The model under review builds one solid part; all positions refer to its coordinate system, in mm. Face numbers are marked on the shaded views. A direction names the side the tool comes from. Give positions to 0.01 mm unless a question says otherwise; leave off trailing zeros. Loops run counter-clockwise (first coordinate to the right, second up) from the corner with the lowest first, then second, coordinate; pieces in that order, holes last. Notation, with made-up numbers: M 40,11 L 90,11 A31 ccw 90,40 Z; hole C 62,78 d3. An arc over 180 degrees is marked long. Return JSON: item names as keys, results as strings.
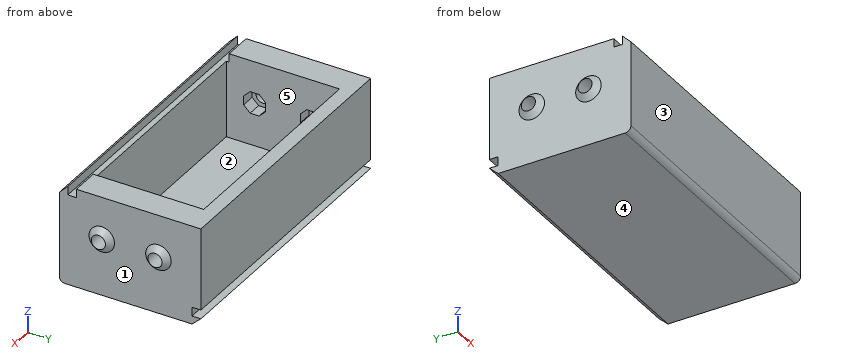
Solid Edge part; units mm, degrees
sketch "Sketch1" plane through (0, 0, 0) normal (-1, 0, 0) x (0, -1, 0)
  line L0 (25, -17.5) -> (25, 17.5)
  line L1 (25, 17.5) -> (-25, 17.5)
  line L2 (-25, 17.5) -> (-25, -17.5)
  line L3 (-25, -17.5) -> (25, -17.5)
extrude "Protrusion1" add sketch "Sketch1" along normal blind 100
sketch "Sketch2" plane through (-50, 0, 17.5) normal (0, 0, 1) x (0, 1, 0)
  line L0 (20, 45) -> (20, -45)
  line L1 (-20, -45) -> (20, -45)
  line L2 (-20, 45) -> (-20, -45)
  line L3 (-20, 45) -> (20, 45)
extrude "Cutout1" cut sketch "Sketch2" against normal blind 30
sketch "Sketch3" plane through (-5, 0, 2.5) normal (-1, 0, 0) x (0, 1, 0)
  line L0 (-20, 15) -> (20, 15)
  line L1 (20, 15) -> (20, -15)
  line L2 (20, -15) -> (-20, -15)
  line L3 (-20, -15) -> (-20, 15)
  line L4 (11.5947, -3.85) -> (8.4053, -3.85)
  line L5 (8.4053, -3.85) -> (6.15, -1.5947)
  line L6 (6.15, -1.5947) -> (6.15, 1.5947)
  line L7 (6.15, 1.5947) -> (8.4053, 3.85)
  line L8 (8.4053, 3.85) -> (11.5947, 3.85)
  line L9 (11.5947, 3.85) -> (13.85, 1.5947)
  line L10 (13.85, 1.5947) -> (13.85, -1.5947)
  line L11 (13.85, -1.5947) -> (11.5947, -3.85)
  line L12 (-11.5947, -3.85) -> (-8.4053, -3.85)
  line L13 (-8.4053, -3.85) -> (-6.15, -1.5947)
  line L14 (-6.15, -1.5947) -> (-6.15, 1.5947)
  line L15 (-6.15, 1.5947) -> (-8.4053, 3.85)
  line L16 (-8.4053, 3.85) -> (-11.5947, 3.85)
  line L17 (-11.5947, 3.85) -> (-13.85, 1.5947)
  line L18 (-13.85, 1.5947) -> (-13.85, -1.5947)
  line L19 (-13.85, -1.5947) -> (-11.5947, -3.85)
extrude "Protrusion2" add sketch "Sketch3" along normal blind 5
sketch "Sketch4" plane through (0, 0, 0) normal (1, 0, 0) x (0, 1, 0)
  circle A0 centre (-10, 2.5) radius 2.5
  circle A1 centre (10, 2.5) radius 2.5
extrude "ExtrudedProtrusion_27" add sketch "Sketch4" along normal blind 5
chamfer "Chamfer_14" distance 2 angle 45 2 edges at (0, 7.5, 2.5) (0, -12.5, 2.5)
sketch "Sketch5" plane through (-100, 0, 0) normal (-1, 0, 0) x (0, -1, 0)
  circle A0 centre (-10, 2.5) radius 2.5
  circle A1 centre (10, 2.5) radius 2.5
extrude "ExtrudedProtrusion_29" add sketch "Sketch5" along normal blind 5
chamfer "Chamfer1" distance 2 angle 45 2 edges at (-100, 10, 0) (-100, -10, 0)
sketch "Sketch6" plane through (-105, 10, 2.5) normal (-1, 0, 0) x (0, -1, 0)
  circle A0 centre (0, 0) radius 2.5
  circle A1 centre (20, 0) radius 2.5
extrude "ExtrudedCutout_41" cut sketch "Sketch6" against normal blind 159
sketch "Sketch7" plane through (-95, 0, 2.5) normal (1, 0, 0) x (0, -1, 0)
  line L0 (-20, 15) -> (20, 15)
  line L1 (20, 15) -> (20, -15)
  line L2 (20, -15) -> (-20, -15)
  line L3 (-20, -15) -> (-20, 15)
  line L4 (-11.5947, 3.85) -> (-8.4053, 3.85)
  line L5 (-8.4053, 3.85) -> (-6.15, 1.5947)
  line L6 (-6.15, 1.5947) -> (-6.15, -1.5947)
  line L7 (-6.15, -1.5947) -> (-8.4053, -3.85)
  line L8 (-8.4053, -3.85) -> (-11.5947, -3.85)
  line L9 (-11.5947, -3.85) -> (-13.85, -1.5947)
  line L10 (-13.85, -1.5947) -> (-13.85, 1.5947)
  line L11 (-13.85, 1.5947) -> (-11.5947, 3.85)
  line L12 (6.15, 1.5947) -> (6.15, -1.5947)
  line L13 (6.15, -1.5947) -> (8.4053, -3.85)
  line L14 (8.4053, -3.85) -> (11.5947, -3.85)
  line L15 (11.5947, -3.85) -> (13.85, -1.5947)
  line L16 (13.85, -1.5947) -> (13.85, 1.5947)
  line L17 (13.85, 1.5947) -> (11.5947, 3.85)
  line L18 (11.5947, 3.85) -> (8.4053, 3.85)
  line L19 (8.4053, 3.85) -> (6.15, 1.5947)
extrude "ExtrudedProtrusion_30" add sketch "Sketch7" along normal blind 5
sketch "Sketch8" plane through (0, 0, 0) normal (1, 0, 0) x (0, -1, 0)
  line L0 (-25, 11.5) -> (-21.85, 11.5)
  line L1 (-21.85, 11.5) -> (-21.85, 14.65)
  line L2 (-21.85, 14.65) -> (-25, 14.65)
  line L3 (-25, 14.65) -> (-21.85, 17.5)
  line L4 (-21.85, 17.5) -> (-21.85, 20.916)
  line L5 (-21.85, 20.916) -> (-29.169, 20.916)
  line L6 (-29.169, 20.916) -> (-29.169, 11.5)
  line L7 (-29.169, 11.5) -> (-25, 11.5)
extrude "Cutout2" cut sketch "Sketch8" against normal blind 112
fillet "Round_8" radius 2 1 edges at (-50, -25, -17.5)
sketch "Sketch9" plane through (0, 0, 0) normal (1, 0, 0) x (0, -1, 0)
  line L0 (22, -14.5) -> (22, -17.5)
  line L1 (25, -14.5) -> (22, -17.5)
  line L2 (25, -14.5) -> (26.5677, -14.5)
  line L3 (26.5677, -14.5) -> (24.562, -20.6312)
  line L4 (24.562, -20.6312) -> (19, -21.06)
  line L5 (19, -14.5) -> (19, -21.06)
  line L6 (19, -14.5) -> (22, -14.5)
extrude "ExtrudedCutout_43" cut sketch "Sketch9" against normal blind 210
1) Wall thickness on L1, parallel to Y at x = -3.5, z = 2.5; L2, parallel to Y at x = -38.5, z = 12.5; L3, parallel to X at y = 13.5, z = 8.5: over which ranges is each line inside the solid? List them lowest first. Write a range as from..to.
From the geometry:
{"L1": "-25..-12.5, -7.5..7.5, 12.5..25", "L2": "-25..-20, 20..25", "L3": "-100..-90, -10..0"}
2) Consider section C-C on z = 11.5. Write out the cut boundary in (x, y).
From the geometry:
{"outline": "M -100,-25 L 0,-25 L 0,25 L -100,25 Z; hole M -90,-20 L -10,-20 L -10,20 L -90,20 Z"}
3) Consider section B-B on x = -17. Write out the cut boundary in (y, z), then the cut area to 3 significant figures.
From the geometry:
{"outline": "M -25,-15.5 A2 ccw -23,-17.5 L 21.85,-17.5 L 25,-14.65 L 21.85,-14.65 L 21.85,-11.5 L 25,-11.5 L 25,17.5 L 20,17.5 L 20,-12.5 L -20,-12.5 L -20,14.5 L -22,14.5 L -22,17.5 L -25,14.5 Z", "area": "524 mm²"}
4) The part is to be moulded in two halves that separate along X. For the marked faces 1, 2 and 3, say which applies: released by +X, released by -X, zero draft, split by the parting line, or undercut.
From the geometry:
{"face 1": "released by +X", "face 2": "undercut", "face 3": "zero draft"}
5) Consider section D-D on y = 4. Write out the cut boundary in (x, z).
From the geometry:
{"outline": "M -100,-17.5 L 0,-17.5 L 0,17.5 L -10,17.5 L -10,-12.5 L -90,-12.5 L -90,17.5 L -100,17.5 Z"}
6) Tool access review of the marked faces 4 and 5: name each direction out of +Z, -Z, +X, -X, +Y, -Y from which nothing blocks a thin tool from reaching the whole face with its end or side.
From the geometry:
{"face 4": "-Z, +X, -X, +Y, -Y", "face 5": "+Z"}
7) Consider section A-A on y = -10. Write out the cut boundary in (x, z).
From the geometry:
{"outline": "M -102,0 L -100,-2 L -100,-17.5 L 0,-17.5 L 0,-2 L 2,0 L -5,0 L -5,-1.35 L -10,-1.35 L -10,-12.5 L -90,-12.5 L -90,-1.35 L -95,-1.35 L -95,0 Z; M -102,5 L -95,5 L -95,6.35 L -90,6.35 L -90,17.5 L -100,17.5 L -100,7 Z; M -10,6.35 L -5,6.35 L -5,5 L 2,5 L 0,7 L 0,17.5 L -10,17.5 Z"}
8) Insertion check: pin 1 (1.6 mm diameter, centred on x = -74.5, y = 23, fed in from -Z); pin 2 (5 mm diameter, centred on x = -45, y = -7.5, fed in from +Z); pin 3 (0.9 mm diameter, centred on x = -67, y = -20.5, fed in from +Z); pin 4 (3 mm diameter, centred on y = 10, z = 2.5, fed in from -X). Each pin has a flat end and moves straight along its axis. Give the tip position at first contact, or say it passes through.
From the geometry:
{"pin 1": "z = -17.18", "pin 2": "z = -12.5", "pin 3": "z = 14.5", "pin 4": "through"}
